```python
from build123d import *

# Parameters (mm, degrees)
SKETCH1_W                  = 180
SKETCH1_H                  = 103
BASE_FLANGE1_DEPTH         = 2
EDGE_FLANGE1_DEPTH         = 180
EDGE_FLANGE1_START         = 2
EDGE_FLANGE1_FLAT_DEPTH    = 2
F_5_1_5_1_DIAMETER_HOLE1_D = 5.1
LPATTERN1_COUNT            = 2
LPATTERN1_PITCH            = 143.6
LPATTERN1_COUNT_DIR2       = 2
LPATTERN1_PITCH_DIR2       = 93.6
M3_TAPPED_HOLE1_D          = 2.5
CUT_EXTRUDE1_DEPTH         = 115.914098352
FILLET1_R                  = 1
BODY_MOVE_COPY1_ANGLE      = 180


# Sheet-metal steps are written as plain solids
with BuildPart() as part:
    # Sketch1 → Base-Flange1 (new body)
    with BuildSketch(Plane(origin=(0, 0, 0), x_dir=(1, 0, 0), z_dir=(0, 1, 0))):
        Rectangle(SKETCH1_W, SKETCH1_H)
    extrude(amount=-BASE_FLANGE1_DEPTH)

    # Edge-Flange1 bend section (across the edge) → Edge-Flange1 (add)
    with BuildSketch(Plane(origin=(90, 0, -53.5), x_dir=(0, 0, 1), z_dir=(-1, 0, 0))):
        with BuildLine():
            Line((-2, 2), (0, 2))
            ThreePointArc((0, 2), (0.585786438, 0.585786438), (2, 0))
            Line((2, 0), (2, -2))
            ThreePointArc((2, -2), (-0.828427125, -0.828427125), (-2, 2))
        make_face()
    extrude(amount=EDGE_FLANGE1_DEPTH)

    # Edge-Flange1 profile (on flange) → Edge-Flange1 flat (add)
    with BuildSketch(Plane(origin=(0, 0, -53.5), x_dir=(-1, 0, 0), z_dir=(0, 0, -1)).offset(EDGE_FLANGE1_START)):
        with BuildLine():
            ThreePointArc((86, 20.3), (83.8, 22.5), (86, 24.7))
            Line((86, 24.7), (90, 24.7))
            Line((90, 24.7), (90, 45))
            Line((90, 45), (-90, 45))
            Line((-90, 45), (-90, 24.7))
            Line((-90, 24.7), (-86, 24.7))
            ThreePointArc((-86, 24.7), (-83.8, 22.5), (-86, 20.3))
            Line((-86, 20.3), (-90, 20.3))
            Line((-90, 20.3), (-90, 2))
            Line((-90, 2), (90, 2))
            Line((90, 2), (90, 20.3))
            Line((90, 20.3), (86, 20.3))
        make_face()
    extrude(amount=-EDGE_FLANGE1_FLAT_DEPTH)

    # Ø5.1 (5.1) Diameter Hole1 (through all)
    with Locations(Plane(origin=(0, -2, 0), x_dir=(-1, 0, 0), z_dir=(0, -1, 0))):
        with Locations((-71.8, -47.3)):
            f_5_1_5_1_diameter_hole1 = Hole(F_5_1_5_1_DIAMETER_HOLE1_D / 2)

    # LPattern1: 5.1 _5.1_ Diameter Hole1 2 × 2
    with Locations(*[(-i * LPATTERN1_PITCH, 0, -j * LPATTERN1_PITCH_DIR2) for i in range(LPATTERN1_COUNT) for j in range(LPATTERN1_COUNT_DIR2) if (i, j) != (0, 0)]):
        add(f_5_1_5_1_diameter_hole1, mode=Mode.SUBTRACT)

    # M3 Tapped Hole1 (through all)
    with Locations(Plane(origin=(0, 0, 0), x_dir=(1, 0, 0), z_dir=(0, 1, 0))):
        with Locations((-85, -29), (85, -29), (-85, 31), (85, 31)):
            Hole(M3_TAPPED_HOLE1_D / 2)

    # Sketch13 → Cut-Extrude1 (cut, through all)
    with BuildSketch(Plane(origin=(0, 0, 0), x_dir=(1, 0, 0), z_dir=(0, 1, 0))):
        with BuildLine():
            Line((-90, 44.2), (-84, 44.2))
            ThreePointArc((-84, 44.2), (-81.8, 42), (-84, 39.8))
            Line((-84, 39.8), (-90, 39.8))
            Line((-90, 39.8), (-90, 44.2))
        make_face()
        with BuildLine():
            Line((-90, -39.8), (-90, -44.2))
            Line((-90, -44.2), (-84, -44.2))
            ThreePointArc((-84, -44.2), (-81.8, -42), (-84, -39.8))
            Line((-84, -39.8), (-90, -39.8))
        make_face()
        with BuildLine():
            Line((90, -44.2), (84, -44.2))
            ThreePointArc((84, -44.2), (81.8, -42), (84, -39.8))
            Line((84, -39.8), (90, -39.8))
            Line((90, -39.8), (90, -44.2))
        make_face()
        with BuildLine():
            Line((90, 39.8), (90, 44.2))
            Line((90, 44.2), (84, 44.2))
            ThreePointArc((84, 44.2), (81.8, 42), (84, 39.8))
            Line((84, 39.8), (90, 39.8))
        make_face()
    extrude(amount=-CUT_EXTRUDE1_DEPTH, mode=Mode.SUBTRACT)

    # Fillet1
    fillet1_edges = [part.edges().sort_by_distance(p)[0] for p in [
        (90, -1, -44.2),
        (90, -1, -39.8),
        (90, -1, 39.8),
        (90, -1, 44.2),
        (-90, -1, 44.2),
        (-90, -1, 39.8),
        (-90, -1, -39.8),
        (-90, -1, -44.2),
        (90, 20.3, -54.5),
        (-90, 20.3, -54.5),
        (-90, 24.7, -54.5),
        (-90, 45, -54.5),
        (90, 45, -54.5),
        (90, 24.7, -54.5),
        (90, -1, 51.5),
        (-90, -1, 51.5),
    ]]
    fillet(fillet1_edges, radius=FILLET1_R)


with BuildPart() as part_1:
    # Body-Move/Copy1: moved
    add(part.part.rotate(Axis((0, 0, 0), (0, 1, 0)), BODY_MOVE_COPY1_ANGLE))


solid = part_1.part
```
The model under review builds one solid part; all positions refer to its coordinate system, in mm. A direction names the side the tool comes from. Give positions to 0.01 mm unless a question says otherwise; leave off trailing zeros. Write each loop counter-clockwise with the first axis right and the second up, starting at its lowest first coordinate (ties: lowest second). Pieces come first, ordered by that corner, then holes. Notation, with made-up numbers: (33.25, -18.75) -> (75.25, -18.75) arc R29 cw to (75.25, 4.25) -> close; hole circle Ø3 at (-21.5, 23). An arc over 180 degrees is marked (long way). Put each result on its own line as item: value.
(1) Tool access review of faces 4 (the cylindrical face through (73.824, -0.986, 44.748)), 5 (the flat face through (1, 0, 1)): name each direction out of +Z, -Z, +X, -X, +Y, -Y from which nothing blocks a thin tool from reaching the whole face with its end or side.
Results are:
face 4: +Y, -Y
face 5: -Z, +X, -X, +Y
(2) We need section D-D, the plane y = 4. Give the boundary of the cut face in (x, z).
Results are:
outline: (-90, 53.5) -> (90, 53.5) -> (90, 55.5) -> (-90, 55.5) -> close
(3) We need section B-B, the plane z = -47.3. Give the boundary of the cut face in (x, y).
Results are:
outline: (-90, -2) -> (-74.35, -2) -> (-74.35, 0) -> (-90, 0) -> close; (-69.25, -2) -> (69.25, -2) -> (69.25, 0) -> (-69.25, 0) -> close; (74.35, -2) -> (90, -2) -> (90, 0) -> (74.35, 0) -> close
(4) We need section C-C, the plane x = 26.5. Give the boundary of the cut face in (y, z).
Results are:
outline: (-2, -51.5) -> (0, -51.5) -> (0, 51.5) arc R2 cw to (2, 53.5) -> (45, 53.5) -> (45, 55.5) -> (2, 55.5) arc R4 ccw to (-2, 51.5) -> close
(5) The part is to be moulded in two halves that separate along X. For faces 1 (the cylindrical face through (-74.156, -0.986, -48.277)), 2 (the flat face through (-90, 7, 54)), 3 (the flat face through (-1, 24, 55.5)), say which applies: pulls with the +X half, pulls with the -X half, needs draft (parallel to the pull), parting line crosses it, or undercut.
Results are:
face 1: undercut
face 2: pulls with the -X half
face 3: needs draft
(6) To check wall thickness, follow probe 1 along Z at (x, y) = (-71.8, -1.45); probe 2 along Z at (x, y) = (-25.5, 28); probe 3 along Y at (x, z) = (-9, 10). State the ranges of each line that lie inside material, in increasing order. Write a range as from..to.
Results are:
probe 1: -51.5..-49.85, -44.75..43.75, 48.85..53.52
probe 2: 53.5..55.5
probe 3: -2..0
(7) For pin 1 Ø2 at (x, z) = (85, 31) entering from +Y; pin 2 Ø0.6 at (x, y) = (-87, -0.5) entering from +Z; pin 3 Ø6 at (x, z) = (71.8, 46.3) entering from +Y; pin 4 Ø2 at (x, y) = (85.5, -1) entering from +Z, all flat-tipped, find the tip position at first contact; note any pin that passes through.
Results are:
pin 1: through
pin 2: z = 54.84
pin 3: y = 0
pin 4: z = 54.96
(8) We need section A-A, the plane x = 71.8. Give the boundary of the cut face in (y, z).
Results are:
outline: (-2, -51.5) -> (0, -51.5) -> (0, -49.85) -> (-2, -49.85) -> close; (-2, -44.75) -> (0, -44.75) -> (0, 43.75) -> (-2, 43.75) -> close; (-2, 48.85) -> (0, 48.85) -> (0, 51.5) arc R2 cw to (2, 53.5) -> (45, 53.5) -> (45, 55.5) -> (2, 55.5) arc R4 ccw to (-2, 51.5) -> close
